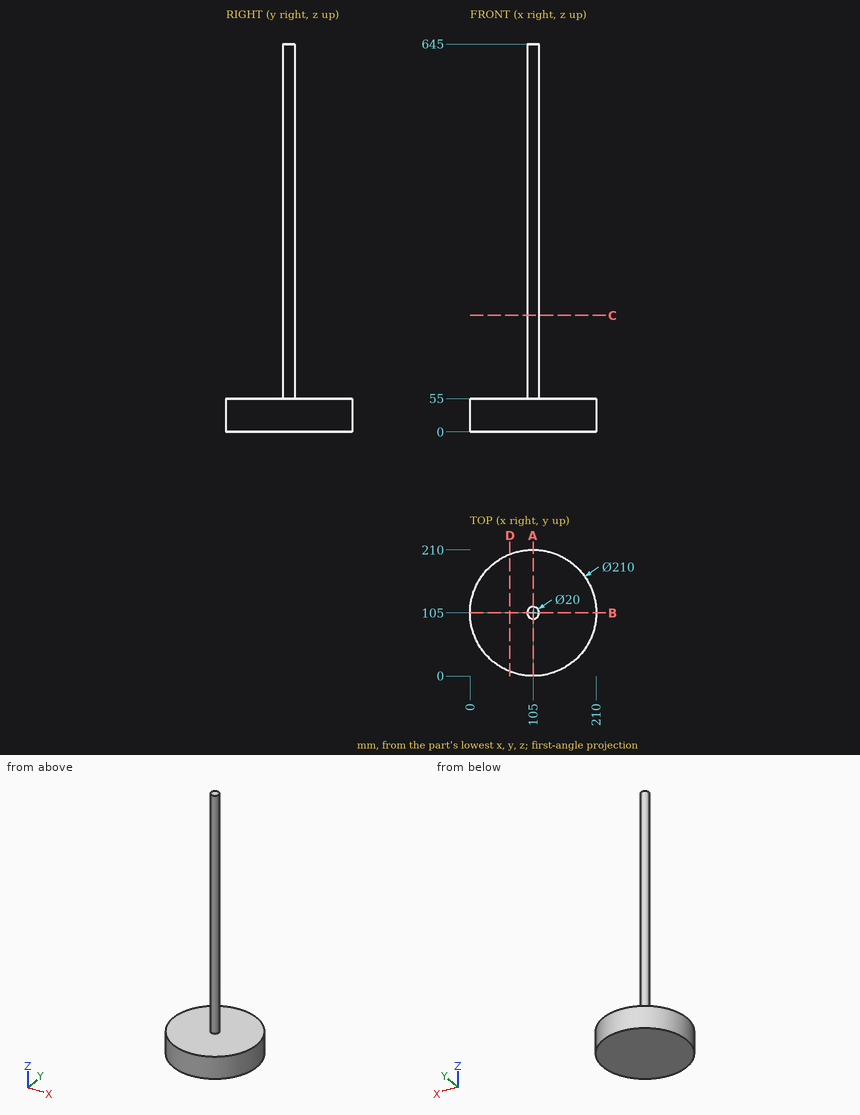
Print and shaded views of the part. All mm, measured from the part's lowest x, y and z. Give positions to 0.01 mm unless a question says otherwise; leave off trailing zeros. Order: outer loops, then holes, each group sorted by start corner. A loop starts at its lowest first (then second) coordinate and runs counter-clockwise, first axis right, second up. Notation, with made-up numbers: (-19.5, 47) - (17.5, 47) arc R21 ccw to (17.5, 67) - close; hole circle Ø1 at (2, -30.75). An arc over 180 degrees is marked (long way). Use a Markdown table: item, result.
1) Probe L1, parallel to Z at x = 122.5, y = 103; L2, parallel to Y at x = 131.5, z = 40.5; L3, parallel to X at y = 112, z = 143.5. List the from-to ranges inside material, lowest first. Write a range as from..to.
Checked values:
| item | result |
|---|---|
| L1 | 0..55 |
| L2 | 3.4..206.6 |
| L3 | 97.86..112.14 |
2) Saw through at C-C on z = 193.5. List the corners of the cut face in (x, y), plus the area to 3 significant figures.
Checked values:
| item | result |
|---|---|
| outline | circle Ø20 at (105, 105) |
| area | 314 mm² |
3) Flat gauge pins, fed straight in: P1, Ø2, axis at x = 75, y = 163, coming from the -Z side; P2, Ø4, axis at x = 125.5, y = 137, coming from the +Z side. Where does each tip first touch, or does it go through?
Checked values:
| item | result |
|---|---|
| P1 | z = 0 |
| P2 | z = 55 |
4) Saw through at A-A on x = 105. List the corners of the cut face in (y, z).
Checked values:
| item | result |
|---|---|
| outline | (0, 0) - (210, 0) - (210, 55) - (115, 55) - (115, 645) - (95, 645) - (95, 55) - (0, 55) - close |
5) Saw through at D-D on x = 66.5. List the corners of the cut face in (y, z).
Checked values:
| item | result |
|---|---|
| outline | (7.31, 0) - (202.69, 0) - (202.69, 55) - (7.31, 55) - close |
